```python
from build123d import *

# Parameters (mm, degrees)
PAD001_DEPTH    = 3
SKETCH006_R     = 4
PAD002_DEPTH    = 7
SKETCH007_R     = 2.25
POCKET002_DEPTH = 6


with BuildPart() as part:
    # Sketch005 → Pad001 (new body, symmetric)
    with BuildSketch(Plane.YZ.offset(-156.5)):
        Polygon((-81.000001, 49), (-81.000001, 41), (-74, 41), (-70, 49), align=None)
    extrude(amount=PAD001_DEPTH, both=True)

    # Sketch006 (on Face1 of Pad001) → Pad002 (join)
    with BuildSketch(Plane(origin=(0, -81.000001, 0), x_dir=(0, 0, -1), z_dir=(0, -1, 0))):
        with Locations((-41.500001, -156.500002)):
            Circle(SKETCH006_R)
    extrude(amount=-PAD002_DEPTH)

    # Sketch007 (on Face7 of Pad002) → Pocket002 (cut)
    with BuildSketch(Plane(origin=(0, -81.000001, 0), x_dir=(0, 0, -1), z_dir=(0, -1, 0))):
        with Locations((-41.500001, -156.500002)):
            Circle(SKETCH007_R)
    extrude(amount=-POCKET002_DEPTH, mode=Mode.SUBTRACT)


solid = part.part
```
Input: part model. Units: mm. Frame: model coordinates. A direction names the side the tool comes from. Give positions to 0.01 mm unless a question says otherwise; leave off trailing zeros. Write each loop counter-clockwise with the first axis right and the second up, starting at its lowest first coordinate (ties: lowest second). Pieces come first, ordered by that corner, then holes. Notation, with made-up numbers: (29.25, 42.5) - (69.25, 42.5) arc R31 ccw to (69.25, 70.5) - close; hole circle Ø5 at (45, 0). An arc over 180 degrees is marked (long way). Write item = value, one per line. Start each with the question number.
1. Section query B-B, the plane y = -75.75. Output: boundary loops of the cut face in (x, z).
2. Access query for faces 1 (the flat face through (-156, -75, 49)), 2 (the flat face through (-156, -75, 42)). Directions: +Z, -Z, +X, -X, +Y, -Y. A direction counts if a zero-diameter tool reaches every point of the face in a straight line with its end or side. Return the directions, or none.
3. First-contact query: pin 1 Ø1 at (y, z) = (-72.5, 42.5) entering from -X; pin 2 Ø4 at (y, z) = (-79.5, 46.5) entering from +X; pin 3 Ø3.5 at (x, z) = (-156.5, 41.5) entering from -Y; pin 4 Ø2.5 at (y, z) = (-73, 44.5) entering from +X. Flat tips, straight axial feed; report the tip coordinate or a pass-through.
4. Mould query, pull axis Z, two halves, no side actions, for faces 3 (the cylindrical face through (-156.6, -77.5, 37.5)), 4 (the flat face through (-156, -81, 45)), 5 (the cylindrical face through (-154.603, -78.042, 40.29)). Classes: released by +Z, released by -Z, zero draft, split by the parting line, or undercut.
5. Section query A-A, the plane z = 41.5. Output: boundary loops of the cut face in (x, y), then the cut area to 3 significant figures.
6. Section query D-D, the plane y = -72. Output: boundary loops of the cut face in (x, z).
7. Ray query, L1, parallel to X at y = -79.8, z = 41.5; L2, parallel to X at y = -75, z = 44.5; L3, parallel to Z at x = -155.75, y = -76.75. Return the intervals inside material, ascending.
Check sheet entries:
q1.outline = (-159.5, 44.15) arc R4 ccw (long way) to (-153.5, 44.15) - (-153.5, 49) - (-159.5, 49) - close; hole circle Ø4.5 at (-156.5, 41.5)
q2.face_1 = +Z, +X, -X, +Y, -Y
q2.face_2 = -Y
q3.pin_1 = through
q3.pin_2 = -153.5
q3.pin_3 = -75
q3.pin_4 = -153.19
q4.face_3 = split by the parting line
q4.face_4 = zero draft
q4.face_5 = undercut
q5.outline = (-160.5, -81) - (-158.75, -81) - (-158.75, -75) - (-154.25, -75) - (-154.25, -81) - (-152.5, -81) - (-152.5, -74) - (-153.5, -74) - (-153.5, -73.75) - (-159.5, -73.75) - (-159.5, -74) - (-160.5, -74) - close
q5.area = 30.5 mm2
q6.outline = (-159.5, 45) - (-153.5, 45) - (-153.5, 49) - (-159.5, 49) - close
q7.L1 = -160.5 to -158.75, -154.25 to -152.5
q7.L2 = -159.5 to -153.5
q7.L3 = 37.57 to 39.38, 43.62 to 49
